Source: CAD feature listing. Evaluate the final solid. Frame: model axes, mm. Give positions to 0.01 mm unless a question says otherwise; leave off trailing zeros. Write each loop counter-clockwise with the first axis right and the second up, starting at its lowest first coordinate (ties: lowest second). Pieces come first, ordered by that corner, then holes. Notation, with made-up numbers: (57, 69.5) -> (110, 69.5) arc R27 cw to (110, 104.5) -> close; hole circle Ø6 at (42, -40). An arc over 180 degrees is marked (long way). Answer as a JSON object with one key per item and string values. Group by question number.
Item 1: First-contact query: pin 1 Ø1 at (x, y) = (107, -65.5) entering from -Z; pin 2 Ø1.5 at (x, z) = (-206.5, 1.5) entering from +Y; pin 3 Ø0.9 at (y, z) = (23.5, 1) entering from +X; pin 4 Ø0.9 at (x, z) = (203, 2) entering from -Y. Flat tips, straight axial feed; report the tip coordinate or a pass-through.
Item 2: Ray query, probe 1 along Y at (x, z) = (173, 1.7). Return the intervals inside material, ascending. Write a range as from..to.
Item 3: Section query B-B on y = -56. Return the cut outline in (x, z), plus the area to 3 significant figures.
Item 4: Section query A-A on z = 0.5. Return the cut outline in (x, y).
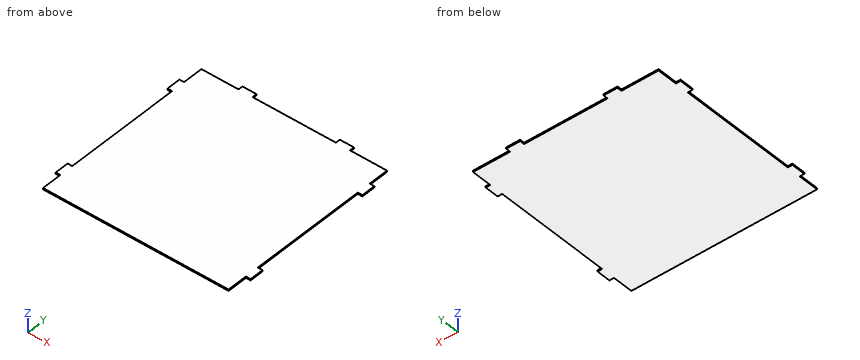
from build123d import *

# Parameters (mm, degrees)
CROQUIS1_W              = 400
CROQUIS1_H              = 400
CROQUIS1_W_2            = 10
CROQUIS1_H_2            = 30
CROQUIS1_W_3            = 30
CROQUIS1_H_3            = 10
SALIENTE_EXTRUIR1_DEPTH = 3


with BuildPart() as part:
    # Croquis1 → Saliente-Extruir1 (new body)
    with BuildSketch(Plane.XY):
        Rectangle(CROQUIS1_W, CROQUIS1_H)
        with Locations((205, 141.243683163)):
            Rectangle(CROQUIS1_W_2, CROQUIS1_H_2)
        with Locations((205, -141.243683163)):
            Rectangle(CROQUIS1_W_2, CROQUIS1_H_2)
        with Locations((-205, -141.243683163)):
            Rectangle(CROQUIS1_W_2, CROQUIS1_H_2)
        with Locations((-205, 141.243683163)):
            Rectangle(CROQUIS1_W_2, CROQUIS1_H_2)
        with Locations((-105, 205)):
            Rectangle(CROQUIS1_W_3, CROQUIS1_H_3)
        with Locations((105, 205)):
            Rectangle(CROQUIS1_W_3, CROQUIS1_H_3)
    extrude(amount=SALIENTE_EXTRUIR1_DEPTH)


solid = part.part
Worked answers:
{
 "1": {"pin 1": "z = 0", "pin 2": "y = 156.24", "pin 3": "x = 200", "pin 4": "y = -156.24"},
 "2": {"probe 1": "-200..200"},
 "3": {"outline": "(-200, 0) -> (200, 0) -> (200, 3) -> (-200, 3) -> close", "area": "1,200 mm^2"},
 "4": {"outline": "(-210, -156.24) -> (-200, -156.24) -> (-200, -200) -> (200, -200) -> (200, -156.24) -> (210, -156.24) -> (210, -126.24) -> (200, -126.24) -> (200, 126.24) -> (210, 126.24) -> (210, 156.24) -> (200, 156.24) -> (200, 200) -> (120, 200) -> (120, 210) -> (90, 210) -> (90, 200) -> (-90, 200) -> (-90, 210) -> (-120, 210) -> (-120, 200) -> (-200, 200) -> (-200, 156.24) -> (-210, 156.24) -> (-210, 126.24) -> (-200, 126.24) -> (-200, -126.24) -> (-210, -126.24) -> close"}
}
